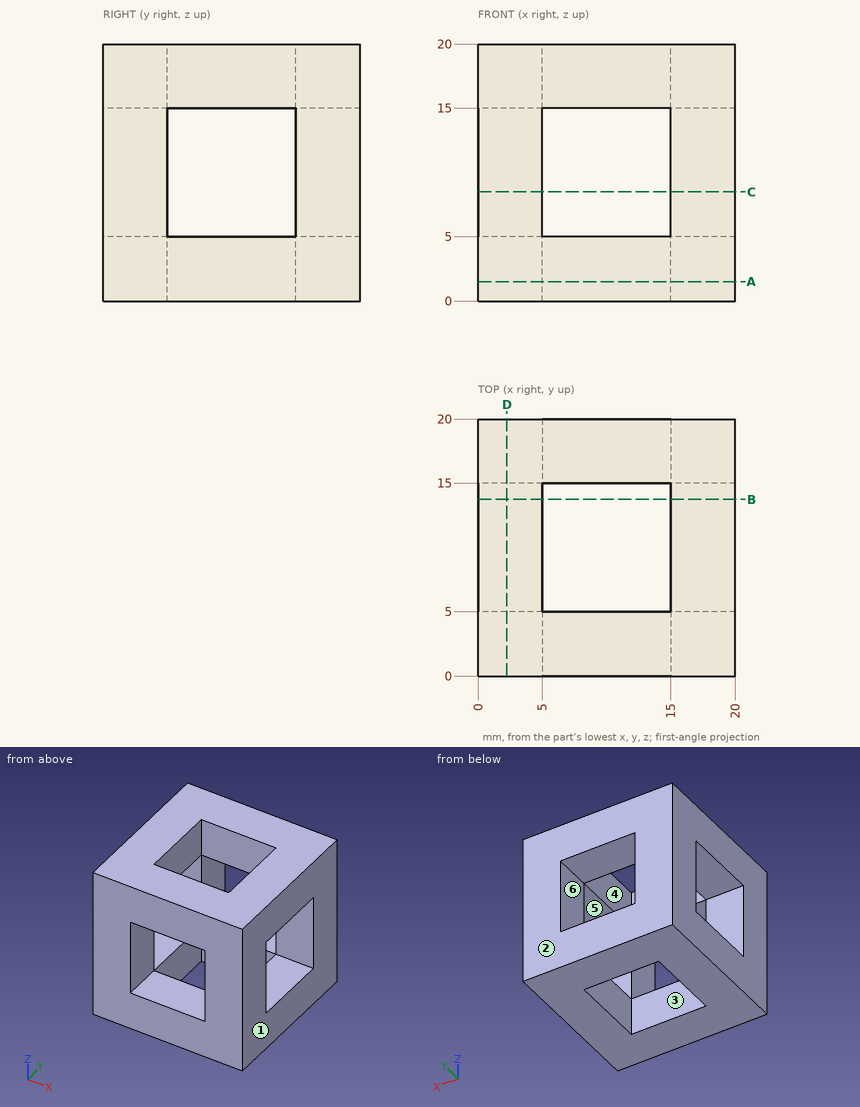
Job drawing, mm, ordinate dimensions from the low corner. One solid piece. A direction names the side the tool comes from. Coordinates: 2 decimals unless noted, no trailing zeros. Loops run counter-clockwise (first coordinate to the right, second up) from the corner with the lowest first, then second, coordinate; pieces in that order, holes last. Notation, with made-up numbers: (78, 31.5) - (117, 31.5) arc R20 ccw to (117, 45.5) - close; hole circle Ø11 at (66, 37). An arc over 180 degrees is marked (long way). Write item = value, one per line. Start each with the question number.
Q1. Cut at B-B, the plane y = 13.75. List the corners of the cut face in (x, z), then the cut area to 3 significant figures.
Q2. Pull direction X, two halves, no side cores. Call the marked faces 1, 2 and 3: pulls with the +X half, pulls with the -X half, needs draft (parallel to the pull), parting line crosses it, or undercut.
Q3. Which spindle directions (+Z, -Z, +X, -X, +Y, -Y) get a long thin tool onto all of the face, cutting with end or side? Do the marked faces 4, 5 and 6. Say none if no direction does.
Q4. Cut at A-A, the plane z = 1.5. List the corners of the cut face in (x, y), then the cut area to 3 significant figures.
Q5. Flat gauge pin, fed straight in: pin 1 Ø2 at (x, z) = (9, 12.5) entering from -Y. Where does the tip first touch, or does it go through?
Q6. Drill centre line: L1, parallel to X at y = 2, z = 12.5. Where is it in solid material? Low to high.
Computed:
q1.outline = (0, 0) - (5, 0) - (5, 5) - (0, 5) - close; (0, 15) - (5, 15) - (5, 20) - (0, 20) - close; (15, 0) - (20, 0) - (20, 5) - (15, 5) - close; (15, 15) - (20, 15) - (20, 20) - (15, 20) - close
q1.area = 100 mm²
q2.face_1 = pulls with the +X half
q2.face_2 = needs draft
q2.face_3 = undercut
q3.face_4 = +Z, -Z
q3.face_5 = +X, -X
q3.face_6 = +Y, -Y
q4.outline = (0, 0) - (20, 0) - (20, 20) - (0, 20) - close; hole (5, 5) - (15, 5) - (15, 15) - (5, 15) - close
q4.area = 300 mm²
q5.pin_1 = through
q6.L1 = 0 to 5, 15 to 20
